Build history of the part. All positions in model axes, mm. Face numbers are marked on the shaded views. A direction names the side the tool comes from. Round coordinates to 2 decimals unless told otherwise and drop trailing zeros. Order: outer loops, then holes, each group sorted by start corner. A loop starts at its lowest first (then second) coordinate and runs counter-clockwise, first axis right, second up. Notation, with made-up numbers: (2.5, 66.5) -> (36.5, 66.5) arc R18 ccw to (36.5, 98.5) -> close; hole circle Ø8 at (38.5, -12.75). An arc over 180 degrees is marked (long way). Answer as a JSON object with one key per item and string values.
Autodesk Inventor part; units mm, degrees
ref_plane "YZ Plane" through (0, 0, 0) normal (1, 0, 0) x (0, 1, 0)
ref_plane "XZ Plane" through (0, 0, 0) normal (0, 1, 0) x (-1, 0, 0)
ref_plane "XY Plane" through (0, 0, 0) normal (0, 0, 1) x (1, 0, 0)
sketch "Sketch1" plane through (0, 0, 0) normal (0, 0, 1) x (1, 0, 0)
  line L0 (0, 0) -> (100, 0)
  line L1 (100, 0) -> (100, 80) construction
  line L2 (100, 80) -> (0, 80)
  line L3 (0, 80) -> (0, 0)
  line L4 (100, 70) -> (90, 80)
  line L5 (100, 10) -> (90, 0)
  line L6 (100, 70) -> (100, 10)
  line L7 (90, 0) -> (0, 0)
  line L8 (90, 80) -> (0, 80)
  dimension "d0" = 100
  dimension "d1" = 80
  dimension "d15" = 10
  dimension "d16" = 10
  dimension "d17" = 10
  dimension "d18" = 10
extrude "Extrusion1" add sketch "Sketch1" along normal blind 40
sketch "Sketch2" plane through (0, 0, 40) normal (0, 0, 1) x (1, 0, 0)
  line L0 (90, 80) -> (0, 80)
  line L1 (100, 70) -> (90, 80)
  line L2 (100, 10) -> (100, 70)
  line L3 (90, 0) -> (100, 10)
  line L4 (0, 0) -> (90, 0)
  line L5 (0, 75) -> (87.9289, 75)
  line L6 (87.9289, 75) -> (95, 67.9289)
  line L7 (95, 67.9289) -> (95, 12.0711)
  line L8 (95, 12.0711) -> (87.9289, 5)
  line L9 (87.9289, 5) -> (0, 5)
  line L10 (0, 80) -> (0, 0)
  line L11 (0, 75) -> (0, 5)
  dimension "d19" = 5
extrude "Extrusion2" cut sketch "Sketch2" against normal blind 35 contours L5 L6 L7 L8 L9 L10
sketch "Sketch3" plane through (0, 0, 0) normal (-1, 0, 0) x (0, 0, 1)
  line L0 (0, 80) -> (40, 80)
  line L1 (0, 0) -> (40, 0)
  line L2 (0, 80) -> (10, 80)
  line L3 (10, 80) -> (10, 50)
  line L4 (10, 50) -> (0, 50)
  line L5 (0, 50) -> (0, 80)
  line L6 (40, 80) -> (40, 0)
  line L7 (0, 80) -> (40, 80)
  line L8 (40, 80) -> (40, 70)
  line L9 (40, 70) -> (0, 70)
  line L10 (0, 70) -> (0, 80)
  line L11 (0, 0) -> (40, 0)
  line L12 (0, 80) -> (40, 80)
  point P0 (20, 0)
  point P1 (20, 80)
  dimension "d7" = 10
  dimension "d8" = 10
  dimension "d11" = 50
extrude "Extrusion3" add sketch "Sketch3" against normal blind 5
sketch "Sketch4" plane through (100, 10, 0) normal (1, 0, 0) x (0, 0, -1)
  circle A0 centre (-40, 30) radius 6
  line L0 (-40, 0) -> (-40, 60)
  point P0 (0, 0)
  dimension "d12" = 12
extrude "Extrusion4" cut sketch "Sketch4" against normal through all
sketch "Sketch5" plane through (0, 0, 5) normal (0, 0, 1) x (1, 0, 0)
  line L0 (74, 75) -> (69, 75)
  line L1 (69, 75) -> (69, 5)
  line L2 (69, 5) -> (74, 5)
  line L3 (74, 5) -> (74, 75)
  line L4 (87.9289, 5) -> (0, 5)
  line L5 (5, 75) -> (87.9289, 75)
  line L6 (95, 67.9289) -> (95, 46)
  point P0 (0, 0)
  dimension "d20" = 5
  dimension "d21" = 21
extrude "Extrusion5" add sketch "Sketch5" along normal blind 35
sketch "Sketch6" plane through (69, 5, 5) normal (-1, 0, 0) x (0, 0, 1)
  line L0 (35, 70) -> (35, 0)
  circle A0 centre (35, 35) radius 3
  line L1 (19.5, 19.5) -> (50.5, 19.5) construction
  line L2 (50.5, 19.5) -> (50.5, 50.5) construction
  line L3 (50.5, 50.5) -> (19.5, 50.5) construction
  line L4 (19.5, 50.5) -> (19.5, 19.5) construction
  line L5 (19.5, 19.5) -> (50.5, 50.5) construction
  line L6 (50.5, 19.5) -> (19.5, 50.5) construction
  circle A1 centre (19.5, 50.5) radius 1.5
  circle A2 centre (19.5, 19.5) radius 1.5
  point P0 (-5, -5)
  dimension "d24" = 6
  dimension "d25" = 31
  dimension "d26" = 31
  dimension "d27" = 3
  dimension "d28" = 3
extrude "Extrusion6" cut sketch "Sketch6" against normal through all
sketch "Sketch7" plane through (69, 5, 5) normal (-1, 0, 0) x (0, 0, 1)
  arc A0 (35, 38) -> (35, 32) centre (35, 35) ccw
  circle A1 centre (35, 35) radius 12.5
  point P0 (-5, -5)
  dimension "d31" = 25
extrude "Extrusion7" cut sketch "Sketch7" against normal blind 2
sketch "Sketch8" plane through (0, 0, 5) normal (0, 0, 1) x (1, 0, 0)
  line L0 (69, 17.5) -> (24, 17.5)
  line L1 (24, 17.5) -> (24, 12.5)
  line L2 (24, 12.5) -> (69, 12.5)
  line L3 (69, 12.5) -> (69, 17.5)
  line L4 (69, 27.5) -> (69, 5)
  line L5 (69, 67.5) -> (24, 67.5)
  line L6 (24, 67.5) -> (24, 62.5)
  line L7 (24, 62.5) -> (69, 62.5)
  line L8 (69, 62.5) -> (69, 67.5)
  line L9 (24, 62.5) -> (24, 17.5) construction
  line L10 (69, 27.5) -> (69, 52.5) construction
  point P0 (0, 0)
  point P1 (69, 15)
  point P2 (24, 40)
  point P3 (69, 40)
  dimension "d34" = 45
  dimension "d35" = 5
  dimension "d36" = 45
  dimension "d37" = 5
  dimension "d38" = 45
extrude "Extrusion8" add sketch "Sketch8" along normal blind 35
sketch "Sketch9" plane through (0, 0, 5) normal (0, 0, 1) x (1, 0, 0)
  line L0 (24, 75) -> (29, 75)
  line L1 (29, 75) -> (29, 5)
  line L2 (29, 5) -> (24, 5)
  line L3 (24, 5) -> (24, 75)
  line L4 (5, 75) -> (69, 75)
  line L5 (69, 5) -> (0, 5)
  point P0 (0, 0)
  point P1 (24, 12.5)
  dimension "d41" = 5
extrude "Extrusion9" add sketch "Sketch9" along normal blind 35
sketch "Sketch10" plane through (0, 0, 40) normal (0, 0, 1) x (1, 0, 0)
  line L0 (29, 17.5) -> (69, 17.5)
  line L1 (24, 5) -> (24, 75)
  line L2 (47, 17.5) -> (24, 17.5)
  line L3 (24, 17.5) -> (24, 5)
  line L4 (24, 5) -> (47, 5)
  line L5 (47, 5) -> (47, 17.5)
  point P0 (0, 0)
  dimension "d44" = 23
extrude "Extrusion10" cut sketch "Sketch10" against normal blind 10
sketch "Sketch11" plane through (0, 0, 5) normal (0, 0, 1) x (1, 0, 0)
  line L0 (34.5, 59.5) -> (37.5, 59.5)
  line L1 (37.5, 59.5) -> (37.5, 20.5)
  line L2 (37.5, 20.5) -> (34.5, 20.5)
  line L3 (34.5, 20.5) -> (34.5, 59.5)
  line L4 (29, 62.5) -> (69, 62.5)
  line L5 (29, 17.5) -> (47, 17.5)
  line L6 (29, 17.5) -> (29, 62.5)
  line L7 (41, 59.5) -> (44, 59.5)
  line L8 (44, 59.5) -> (44, 20.5)
  line L9 (44, 20.5) -> (41, 20.5)
  line L10 (41, 20.5) -> (41, 59.5)
  line L11 (47.5, 59.5) -> (50.5, 59.5)
  line L12 (50.5, 59.5) -> (50.5, 20.5)
  line L13 (50.5, 20.5) -> (47.5, 20.5)
  line L14 (47.5, 20.5) -> (47.5, 59.5)
  line L15 (54, 59.5) -> (57, 59.5)
  line L16 (57, 59.5) -> (57, 20.5)
  line L17 (57, 20.5) -> (54, 20.5)
  line L18 (54, 20.5) -> (54, 59.5)
  line L19 (60.5, 59.5) -> (63.5, 59.5)
  line L20 (63.5, 59.5) -> (63.5, 20.5)
  line L21 (63.5, 20.5) -> (60.5, 20.5)
  line L22 (60.5, 20.5) -> (60.5, 59.5)
  point P0 (0, 0)
  dimension "d47" = 3
  dimension "d48" = 3
  dimension "d49" = 3
  dimension "d50" = 5.5
  dimension "d53" = 6.5
extrude "Extrusion11" cut sketch "Sketch11" against normal through all
sketch "Sketch12" plane through (0, 0, 0) normal (0, -1, 0) x (1, 0, 0)
  circle A0 centre (45, 40) radius 6
  line L0 (0, 40) -> (90, 40)
  point P0 (0, 0)
  dimension "d60" = 12
extrude "Extrusion12" cut sketch "Sketch12" against normal blind 5
properties part number "FA001" material "ABS Plastic"
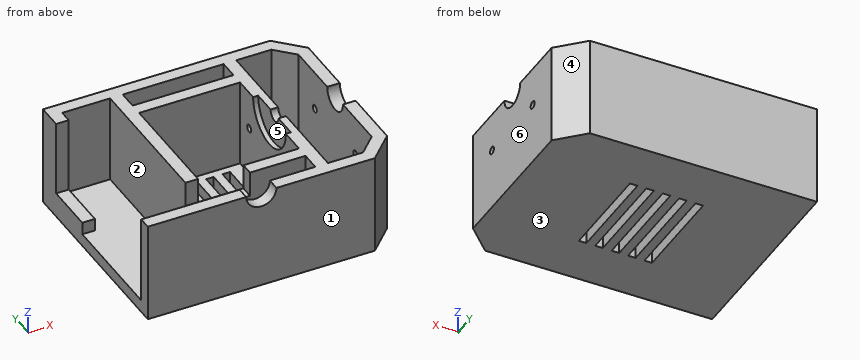
1) Cut at B-B, the plane x = 10. Give the cut face in (y, z).
Checked values:
{"outline": "(0, 0) -> (80, 0) -> (80, 40) -> (75, 40) -> (75, 5) -> (5, 5) -> (5, 40) -> (0, 40) -> close"}
2) Cut at A-A, the plane z = 15.5. Count the separate pieces of the cut face and the enclosed holes in it, plus the area to 4 significant figures.
Checked values:
{"separate pieces": "1", "enclosed holes": "4", "area": "2,425 mm²"}
3) Probe L1, parallel to X at y = 52.5, z = 21; L2, parallel to X at y = 43, z = 30.5; L3, parallel to Y at x = 59.5, z = 25. List the from-to ranges inside material, lowest first. Write a range as from..to.
Checked values:
{"L1": "x = 24..29, 69..74, 95..100", "L2": "x = 24..29, 71..74, 95..100", "L3": "y = 0..5, 12.5..17.5, 62.5..67.5, 75..80"}
4) Pull direction Y, two halves, no side cores. Call the marked faces 1, 2, 3 and 4: pulls with the +Y half, pulls with the -Y half, needs draft (parallel to the pull), parting line crosses it, or undercut.
Checked values:
{"face 1": "pulls with the -Y half", "face 2": "undercut", "face 3": "needs draft", "face 4": "pulls with the +Y half"}
5) Flat gauge pins, fed straight in: pin 1 Ø5.5 at (x, y) = (2, 57.5) entering from +Z; pin 2 Ø17.5 at (y, z) = (39.5, 22) entering from -X; pin 3 Ø12 at (x, y) = (7, 22.5) entering from +Z. Where does each tip first touch, or does it go through?
Checked values:
{"pin 1": "stops at z = 10", "pin 2": "stops at x = 24", "pin 3": "stops at z = 5"}
6) Which spindle directions (+Z, -Z, +X, -X, +Y, -Y) get a long thin tool onto all of the face, cutting with end or side? Do the marked faces 5 and 6. Say none if no direction does.
Checked values:
{"face 5": "+Z", "face 6": "+Z, -Z, +X, +Y, -Y"}
